Model file for the job. Use its own axes, mm. A direction names the side the tool comes from. Give positions to 0.01 mm unless a question says otherwise; leave off trailing zeros. Order: outer loops, then holes, each group sorted by start corner. A loop starts at its lowest first (then second) coordinate and runs counter-clockwise, first axis right, second up. Notation, with made-up numbers: (64.5, 64) -> (102.5, 64) arc R25 cw to (102.5, 97) -> close; hole circle Ø4 at (43.5, 3.25). An arc over 180 degrees is marked (long way). Use CSV: the item, a comma, the result in double quotes. Start each with the question number.
1. Drop flat-ended pins along their axis: pin 1 (19 mm diameter, centred on y = 14.5, z = -21.5, fed in from -X); pin 2 (8 mm diameter, centred on x = 21, y = 25.5, fed in from +Z); pin 3 (15 mm diameter, centred on x = 58, z = -3, fed in from +Y); pin 4 (12 mm diameter, centred on x = 18.5, y = 64.5, fed in from +Z). Give the stop position or say it passes through.
2. Cut at A-A on y = 11.5. List the corners of the cut face in (x, z), then the cut area to 3 significant figures.
3. Pull direction Z, two halves, no side cores. Call faces 6 (the flat face through (1, 45, -26)), 7 (the flat face through (31, 22, 6)), 8 (the flat face through (-13, 70, -8)): released by +Z, released by -Z, zero draft, split by the parting line, or undercut.
4. Cut at B-B on z = 0. List the corners of the cut face in (x, y).
5. Cut at D-D on y = 59. List the corners of the cut face in (x, z).
6. Wall check: line 1 (Z direction, x = -60, y = 10.25); line 2 (Y direction, x = 19, z = -13); line 3 (Y direction, x = 0, z = 19). Give the ranges that are in metal, low to high. Write a range as from..to.
7. 3-axis set-ups, long thin cutter, end or side, ignore diameter. For faces 1 (the cylindrical face through (7.509, 62.255, 23.846)), 2 (the flat face through (45, 30, 0)), 3 (the flat face through (35, 15, -18)), 4 (the flat face through (-60, 15, 0)), 5 (the flat face through (-35, 15, 18)): which of +Z, -Z, +X, -X, +Y, -Y reach the whole face in a straight line?
8. Cut at C-C on x = 0. List the corners of the cut face in (y, z).
```python
from build123d import *

# Parameters (mm, degrees)
BOSS_EXTRUDE1_DEPTH     = 30
BOSS_EXTRUDE2_DEPTH     = 6
SKETCH3_R               = 5.510010548
CUT_EXTRUDE1_DEPTH      = 87.168439698
FILLET1_R               = 10
SKETCH4_R               = 7
CUT_EXTRUDE2_DEPTH      = 42
SKETCH5_R               = 25
BOSS_EXTRUDE3_DEPTH     = 35
SKETCH6_R               = 20
CUT_EXTRUDE3_DEPTH      = 10
SKETCH8_R               = 10
CUT_EXTRUDE4_DEPTH      = 40
CUT_EXTRUDE4_DRAFT      = 7
CUT_EXTRUDE5_DEPTH      = 114.688170009
CUT_EXTRUDE5_DEPTH_BACK = 114.688170009
SKETCH9_R               = 5


with BuildPart() as part:
    # Sketch1 → Boss-Extrude1 (new, symmetric)
    with BuildSketch(Plane.XY):
        Polygon((-45, 15), (-75, 15), (-75, 0), (-35, 0), (-35, 30), (35, 30), (35, 0), (75, 0), (75, 15), (45, 15), (45, 45), (-45, 45), align=None)
    extrude(amount=BOSS_EXTRUDE1_DEPTH, both=True)

    # Sketch2 → Boss-Extrude2 (add, symmetric)
    with BuildSketch(Plane.XY):
        Polygon((20, 30), (35, 0), (35, 30), align=None)
        Polygon((-35, 0), (-20, 30), (-35, 30), align=None)
    extrude(amount=BOSS_EXTRUDE2_DEPTH, both=True)

    # Sketch3 → Cut-Extrude1 (cut, through all)
    with BuildSketch(Plane(origin=(0, 15, 0), x_dir=(1, 0, 0), z_dir=(0, 1, 0))):
        with Locations(Location((-60, 15, 0), (0, 0, 180))):
            Circle(SKETCH3_R)
        with Locations(Location((-60, -15, 0), (0, 0, 180))):
            Circle(SKETCH3_R)
    extrude(amount=-CUT_EXTRUDE1_DEPTH, mode=Mode.SUBTRACT)

    # Fillet1
    fillet1_edges = [part.edges().sort_by_distance(p)[0] for p in [
        (-75, 7.5, -30),
        (-75, 7.5, 30),
    ]]
    fillet(fillet1_edges, radius=FILLET1_R)

    # Sketch4 → Cut-Extrude2 (cut)
    with BuildSketch(Plane(origin=(0, 15, 0), x_dir=(1, 0, 0), z_dir=(0, 1, 0))):
        with Locations((75, 0)):
            Circle(SKETCH4_R)
    extrude(amount=-CUT_EXTRUDE2_DEPTH, mode=Mode.SUBTRACT)

    # Sketch5 → Boss-Extrude3 (add)
    with BuildSketch(Plane(origin=(0, 45, 0), x_dir=(1, 0, 0), z_dir=(0, 1, 0))):
        with Locations(Location((0, 0, 0), (0, 0, 270))):
            Circle(SKETCH5_R)
    extrude(amount=BOSS_EXTRUDE3_DEPTH)

    # Sketch6 → Cut-Extrude3 (cut)
    with BuildSketch(Plane(origin=(0, 80, 0), x_dir=(1, 0, 0), z_dir=(0, 1, 0))):
        with Locations(Location((0, 0, 0), (0, 0, 270))):
            Circle(SKETCH6_R)
    extrude(amount=-CUT_EXTRUDE3_DEPTH, mode=Mode.SUBTRACT)


with BuildPart() as cut_extrude4_tool:
    # Sketch8 → Cut-Extrude4 (with draft: the straight prism first)
    with BuildSketch(Plane.XZ.offset(-30)):
        Circle(SKETCH8_R)
    extrude(amount=-CUT_EXTRUDE4_DEPTH)
    # Cut-Extrude4: the draft: its side faces are tilted about the plane it starts from
    cut_extrude4_sides = [cut_extrude4_tool.faces().sort_by_distance(p)[0] for p in [
        (-10, 50, 0),
    ]]
    draft(cut_extrude4_sides, Plane.XZ.offset(-30), CUT_EXTRUDE4_DRAFT)


with BuildPart() as part_1:
    add(part.part)

    # Cut-Extrude4: cut by cut_extrude4_tool
    add(cut_extrude4_tool.part, mode=Mode.SUBTRACT)

    # Sketch9 → Cut-Extrude5 (cut, two sides: drawn at the far end of the back side and taken through both)
    with BuildSketch(Plane.XY.offset(-CUT_EXTRUDE5_DEPTH_BACK)):
        with Locations((0, 59)):
            Circle(SKETCH9_R)
    extrude(amount=CUT_EXTRUDE5_DEPTH + CUT_EXTRUDE5_DEPTH_BACK, mode=Mode.SUBTRACT)


solid = part_1.part
```
Verdict:
1,pin 1,"x = -75"
1,pin 2,"z = 6"
1,pin 3,"y = 15"
1,pin 4,"z = 21.65"
2,outline,"(-75, -20) arc R10 ccw to (-65, -30) -> (-35, -30) -> (-35, -6) -> (-29.25, -6) -> (-29.25, 6) -> (-35, 6) -> (-35, 30) -> (-65, 30) arc R10 ccw to (-75, 20) -> close; (29.25, -6) -> (35, -6) -> (35, -30) -> (75, -30) -> (75, -7) arc R7 cw to (75, 7) -> (75, 30) -> (35, 30) -> (35, 6) -> (29.25, 6) -> close; hole circle Ø11.02 at (-60, -15); hole circle Ø11.02 at (-60, 15)"
2,area,"4,630 mm^2"
3,face 6,"zero draft"
3,face 7,"released by +Z"
3,face 8,"undercut"
4,outline,"(-75, 0) -> (-35, 0) -> (-20, 30) -> (-10, 30) -> (-14.91, 70) -> (-20, 70) -> (-20, 80) -> (-25, 80) -> (-25, 45) -> (-45, 45) -> (-45, 15) -> (-75, 15) -> close; (10, 30) -> (20, 30) -> (35, 0) -> (68, 0) -> (68, 15) -> (45, 15) -> (45, 45) -> (25, 45) -> (25, 80) -> (20, 80) -> (20, 70) -> (14.91, 70) -> close"
5,outline,"(-5, -24.49) -> (-5, -12.61) arc R13.56 cw to (-5, 12.61) -> (-5, 24.49) arc R25 ccw to start; (5, -24.49) arc R25 ccw to (5, 24.49) -> (5, 12.61) arc R13.56 cw to (5, -12.61) -> close"
6,line 1,"-30..-20.51, -9.49..9.49, 20.51..30"
6,line 2,"30..80"
6,line 3,"30..54, 64..70"
7,face 1,"+Y"
7,face 2,"+Z, -Z, +X, +Y"
7,face 3,"-Z, -Y"
7,face 4,"+Z, -Z, -X, +Y"
7,face 5,"+Z, -Y"
8,outline,"(30, -30) -> (45, -30) -> (45, -25) -> (54, -25) -> (54, -12.95) -> (30, -10) -> close; (30, 10) -> (54, 12.95) -> (54, 25) -> (45, 25) -> (45, 30) -> (30, 30) -> close; (64, -25) -> (80, -25) -> (80, -20) -> (70, -20) -> (70, -14.91) -> (64, -14.17) -> close; (64, 14.17) -> (70, 14.91) -> (70, 20) -> (80, 20) -> (80, 25) -> (64, 25) -> close"
